```python
from build123d import *

# Parameters (mm, degrees)
SKETCH1_W           = 40
SKETCH1_H           = 28
SKETCH1_R           = 2.4
SKETCH1_W_2         = 12
SKETCH1_H_2         = 18.5
BOSS_EXTRUDE1_DEPTH = 5
FILLET1_R           = 3


with BuildPart() as part:
    # Sketch1 → Boss-Extrude1 (new body)
    with BuildSketch(Plane.XY):
        Rectangle(SKETCH1_W, SKETCH1_H)
        with Locations((-10, 8)):
            Circle(SKETCH1_R, mode=Mode.SUBTRACT)
        with Locations((-10, -8)):
            Circle(SKETCH1_R, mode=Mode.SUBTRACT)
        with Locations((10, 0)):
            Rectangle(SKETCH1_W_2, SKETCH1_H_2, mode=Mode.SUBTRACT)
    extrude(amount=BOSS_EXTRUDE1_DEPTH)

    # Fillet1
    fillet1_edges = [part.edges().sort_by_distance(p)[0] for p in [
        (20, -14, 2.5),
        (-20, -14, 2.5),
        (-20, 14, 2.5),
        (20, 14, 2.5),
    ]]
    fillet(fillet1_edges, radius=FILLET1_R)


solid = part.part
```
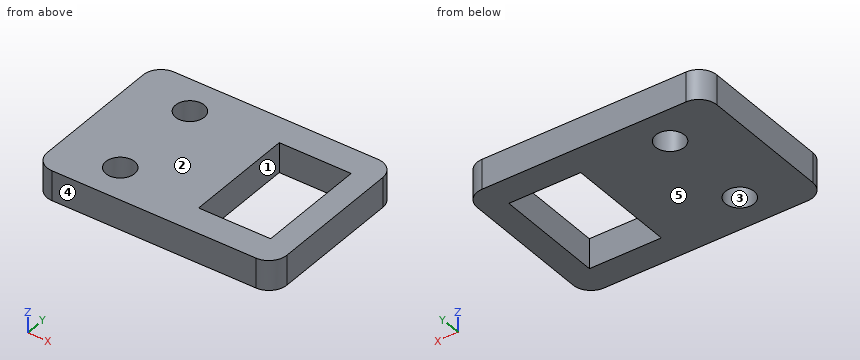
CAD build for the part. Positions are in the model's coordinates, mm. Face numbers are marked on the shaded views. A direction names the side the tool comes from. Give positions to 0.01 mm unless a question says otherwise; leave off trailing zeros. Loops run counter-clockwise (first coordinate to the right, second up) from the corner with the lowest first, then second, coordinate; pieces in that order, holes last. Notation, with made-up numbers: M 2,68 L 26,68 A29 ccw 26,92 Z; hole C 15,-5 d4. An arc over 180 degrees is marked long. Use one line per item in the form item = value.
Item 1: Which spindle directions (+Z, -Z, +X, -X, +Y, -Y) get a long thin tool onto all of the face, cutting with end or side? Do the marked faces 1 and 2. Say none if no direction does.
Determined:
face_1 = +Z, -Z
face_2 = +Z, +X, -X, +Y, -Y
Item 2: Slice it at C-C (y = 4.75). List the corners of the cut face in (x, z).
Determined:
outline = M -20,0 L 4,0 L 4,5 L -20,5 Z; M 16,0 L 20,0 L 20,5 L 16,5 Z
Item 3: Two-plate mould, pull along Y, no slides. Class the marked faces 3, 4 and 5: pulls with the +Y half, pulls with the -Y half, needs draft (parallel to the pull), parting line crosses it, or undercut.
Determined:
face_3 = undercut
face_4 = pulls with the -Y half
face_5 = needs draft
Item 4: Slice it at B-B (y = 8). List the corners of the cut face in (x, z), plus the area to 3 significant figures.
Determined:
outline = M -20,0 L -12.4,0 L -12.4,5 L -20,5 Z; M -7.6,0 L 4,0 L 4,5 L -7.6,5 Z; M 16,0 L 20,0 L 20,5 L 16,5 Z
area = 116 mm2
Item 5: Drill centre lines: probe 1 along Y at (x, z) = (-10, 2.45); probe 2 along Y at (x, z) = (6.5, 1.2); probe 3 along Y at (x, z) = (-11, 3.25). Where is each one in solid material? Low to high. Write a range as from..to.
Determined:
probe_1 = -14..-10.4, -5.6..5.6, 10.4..14
probe_2 = -14..-9.25, 9.25..14
probe_3 = -14..-10.18, -5.82..5.82, 10.18..14
Item 6: Slice it at A-A (x = 6). List the corners of the cut face in (y, z).
Determined:
outline = M -14,0 L -9.25,0 L -9.25,5 L -14,5 Z; M 9.25,0 L 14,0 L 14,5 L 9.25,5 Z
Item 7: Slice it at D-D (z = 1.55). List the corners of the cut face in (x, y), plus the area to 3 significant figures.
Determined:
outline = M -20,-11 A3 ccw -17,-14 L 17,-14 A3 ccw 20,-11 L 20,11 A3 ccw 17,14 L -17,14 A3 ccw -20,11 Z; hole C -10,-8 d4.8; hole C -10,8 d4.8; hole M 4,-9.25 L 16,-9.25 L 16,9.25 L 4,9.25 Z
area = 854 mm2
